CAD build for the part. Positions are in the model's coordinates, mm. A direction names the side the tool comes from. Give positions to 0.01 mm unless a question says otherwise; leave off trailing zeros. Write each loop counter-clockwise with the first axis right and the second up, starting at its lowest first coordinate (ties: lowest second). Pieces come first, ordered by that corner, then holes. Notation, with made-up numbers: (27, 32.5) - (65, 32.5) arc R12 ccw to (65, 40.5) - close; hole circle Ø6 at (80.25, 40). An arc over 180 degrees is marked (long way). Write item = value, one per line. Start each with the question number.
```python
from build123d import *

# Parameters (mm, degrees)
F0_W     = 101.6
F0_H     = 76.2
F1_DEPTH = 25.4
F3_DEPTH = 25.4
F5_DEPTH = 25.4


with BuildPart() as f1:
    # F0 (on Top) → F1 (new body)
    with BuildSketch(Plane.XY):
        with Locations((-12.35143, -30.653376)):
            Rectangle(F0_W, F0_H)
    extrude(amount=F1_DEPTH)

    # F2 (on face) → F3 (join)
    with BuildSketch(Plane.XY.offset(25.4)):
        Polygon((-63.15143, -68.753376), (-12.35143, 7.446624), (-63.15143, 7.446624), align=None)
    extrude(amount=F3_DEPTH)

    # F4 (on face) → F5 (join)
    with BuildSketch(Plane.XY.offset(25.4)):
        Polygon((38.44857, -30.653376), (13.04857, -68.753376), (38.44857, -68.753376), align=None)
    extrude(amount=F5_DEPTH)


solid = f1.part
```
1. Cut at C-C (x = -7). Give the cut face in (y, z).
2. Tool access for faces 5 (the flat face through (-44, -22, 50.8)), 6 (the flat face through (-2, -30, 25.4)), 7 (the flat face through (-38.11, -31.19, 37.92)): list every direction of +Z, -Z, +X, -X, +Y, -Y with a clear straight run to the whole face (end or side of a thin tool).
3. Mould opens along X. For faces 1 (the flat face through (-23, 7.447, 19)), 2 (the flat face through (38.449, -40, 19)), 3 (the flat face through (-63.151, -30, 25)), 4 (the flat face through (25.926, -49.437, 37.922)) say: +X half, -X half, draft (parallel to the pull), parting line (faces both ways), or undercut.
4. Cut at D-D (x = 26.5). Give the cut face in (y, z).
5. Cut at A-A (z = 43.5). Give the cut face in (x, y).
6. Cut at B-B (y = -53.5). Give the cut face in (x, z), then the cut area to 3 significant figures.
7. Wall check: line 1 along Z through (x, y) = (-30.5, -60); line 2 along X through (y, z) = (-34, 37); line 3 along Y through (x, z) = (-17.5, 30). Give the ranges that are in metal, low to high.
8. Pin check, flat tips, straight feed: pin 1 Ø6 at (x, z) = (-9, 42) entering from +Y; pin 2 Ø5 at (x, z) = (14.5, 44) entering from +Y; pin 3 Ø8 at (y, z) = (-20.5, 33) entering from +X; pin 4 Ø10 at (x, y) = (-2, -60) entering from +Z. Stop position of each tip, or through.
Output:
q1.outline = (-68.75, 0) - (7.45, 0) - (7.45, 25.4) - (-68.75, 25.4) - close
q2.face_5 = +Z, +X, -X, +Y, -Y
q2.face_6 = +Z
q2.face_7 = +Z, -Y
q3.face_1 = draft
q3.face_2 = +X half
q3.face_3 = -X half
q3.face_4 = undercut
q4.outline = (-68.75, 0) - (7.45, 0) - (7.45, 25.4) - (-48.58, 25.4) - (-48.58, 50.8) - (-68.75, 50.8) - close
q5.outline = (-63.15, -68.75) - (-12.35, 7.45) - (-63.15, 7.45) - close; (13.05, -68.75) - (38.45, -68.75) - (38.45, -30.65) - close
q6.outline = (-63.15, 0) - (38.45, 0) - (38.45, 50.8) - (23.22, 50.8) - (23.22, 25.4) - (-52.98, 25.4) - (-52.98, 50.8) - (-63.15, 50.8) - close
q6.area = 3,230 mm2
q7.line_1 = 0 to 25.4
q7.line_2 = -63.15 to -39.98, 36.22 to 38.45
q7.line_3 = -0.28 to 7.45
q8.pin_1 = through
q8.pin_2 = -62.83
q8.pin_3 = -28.32
q8.pin_4 = 25.4
